from build123d import *

# Parameters (mm, degrees)
F0_W     = 20
F0_H     = 20
F0_W_2   = 4
F0_H_2   = 4
F0_R     = 1.6
F1_DEPTH = 10
F0_W_3   = 24
F0_H_3   = 24
F2_DEPTH = 2
F3_DEPTH = 5
F5_R     = 5
F6_R     = 5
F7_R     = 1


# Not quite as in the source:
# - the program builds the solid bodies; features that only make, move or delete a surface that nothing else refers to are left out


with BuildPart() as f1:
    # F0 (on Top) → F1 (new body)
    with BuildSketch(Plane.XY):
        Rectangle(F0_W, F0_H)
        Rectangle(F0_W_2, F0_H_2, mode=Mode.SUBTRACT)
        Rectangle(F0_W_2, F0_H_2)
        Circle(F0_R, mode=Mode.SUBTRACT)
        Circle(F0_R)
    extrude(amount=F1_DEPTH)

    # F0 (on Top) → F2 (join)
    with BuildSketch(Plane.XY):
        Rectangle(F0_W_3, F0_H_3)
        Rectangle(F0_W, F0_H, mode=Mode.SUBTRACT)
    extrude(amount=F2_DEPTH)

    # F0 (on Top) → F3 (join)
    with BuildSketch(Plane.XY):
        Rectangle(F0_W_2, F0_H_2)
        Circle(F0_R, mode=Mode.SUBTRACT)
        Circle(F0_R)
    extrude(amount=-F3_DEPTH)

    # F5
    f5_edges = [f1.edges().sort_by_distance(p)[0] for p in [
        (-10, -10, 6),
    ]]
    fillet(f5_edges, radius=F5_R)

    # F6
    f6_edges = [f1.edges().sort_by_distance(p)[0] for p in [
        (10, -10, 6),
        (10, 10, 6),
        (-10, 10, 6),
    ]]
    fillet(f6_edges, radius=F6_R)

    # F7
    f7_edges = [f1.edges().sort_by_distance(p)[0] for p in [
        (2, 2, -2.5),
        (2, -2, -2.5),
        (-2, -2, -2.5),
        (-2, 2, -2.5),
    ]]
    fillet(f7_edges, radius=F7_R)


solid = f1.part
Check sheet for the modelled part. Datum: model origin and axes. Units: mm. A direction names the side the tool comes from. Give positions to 0.01 mm unless a question says otherwise; leave off trailing zeros. Loops run counter-clockwise (first coordinate to the right, second up) from the corner with the lowest first, then second, coordinate; pieces in that order, holes last. Notation, with made-up numbers: M 27,17 L 46,17 A18 cw 46,48 Z; hole C 37.5,58 d6. An arc over 180 degrees is marked long. Return JSON: item names as keys, results as strings. Group by question number.
1. Tool access check on faces 1 (the flat face through (0, 2, -2)), 2 (the flat face through (10, 0, 6)), 3 (the flat face through (0, -2, -2)), 4 (the cylindrical face through (-8, -9, 6)), 5 (the flat face through (-2, 0, -2)). Record the directions out of +Z, -Z, +X, -X, +Y, -Y that give a thin tool (end or side, any length) a straight path to the whole face; none if there is none.
2. Thickness scan on L1, parallel to Z at x = 2.75, y = 11.25; L2, parallel to Z at x = 7.5, y = 4; L3, parallel to X at y = -1, z = 9.25. Record the ranges inside material, lowest first.
3. Go/stop test with flat-tipped pins: pin 1 (1 mm diameter, centred on x = 2, y = 2.5, fed in from -Z); pin 2 (4 mm diameter, centred on x = -1, z = 8, fed in from -Y); pin 3 (0.6 mm diameter, centred on x = 0.5, z = -2.5, fed in from -Y); pin 4 (8 mm diameter, centred on y = -0.5, z = -2.5, fed in from +X). Record where each tip stops, or that it passes through.
4. Cross-section at D-D on x = 10.5. Record the boundary of the cut face in (y, z), plus the area to 3 significant figures.
5. Cross-section at B-B on y = 3. Record the boundary of the cut face in (x, z), plus the area to 3 significant figures.
6. Cross-section at A-A on z = -2.25. Record the boundary of the cut face in (x, y).
7. Cross-section at C-C on y = -0.25. Record the boundary of the cut face in (x, z).
Return value:
{
 "1": {"face 1": "-Z, +X, -X, +Y", "face 2": "+Z, +X, +Y, -Y", "face 3": "-Z, +X, -X, -Y", "face 4": "+Z, -X, -Y", "face 5": "-Z, -X, +Y, -Y"},
 "2": {"L1": "0 to 2", "L2": "0 to 10", "L3": "-10 to 10"},
 "3": {"pin 1": "z = 0", "pin 2": "y = -10", "pin 3": "y = -2", "pin 4": "x = 12"},
 "4": {"outline": "M -12,0 L 12,0 L 12,2 L -12,2 Z", "area": "48.0 mm^2"},
 "5": {"outline": "M -12,0 L 12,0 L 12,2 L 10,2 L 10,10 L -10,10 L -10,2 L -12,2 Z", "area": "208 mm^2"},
 "6": {"outline": "M -2,-1 A1 ccw -1,-2 L 1,-2 A1 ccw 2,-1 L 2,1 A1 ccw 1,2 L -1,2 A1 ccw -2,1 Z"},
 "7": {"outline": "M -12,0 L -2,0 L -2,-5 L 2,-5 L 2,0 L 12,0 L 12,2 L 10,2 L 10,10 L -10,10 L -10,2 L -12,2 Z"}
}
